from build123d import *

# Parameters (mm, degrees)
ESBO_O1_W                = 150
ESBO_O1_H                = 55
RESSALTO_EXTRUS_O1_DEPTH = 45
FILETE1_R                = 8
ESBO_O2_R                = 3.81
RESSALTO_EXTRUS_O2_DEPTH = 16.806
ESBO_O4_R                = 3.81
RESSALTO_EXTRUS_O3_DEPTH = 16.806


with BuildPart() as part:
    # Esboço1 → Ressalto-extrusão1 (new body)
    with BuildSketch(Plane(origin=(0, 0, 0), x_dir=(1, 0, 0), z_dir=(0, 1, 0))):
        Rectangle(ESBO_O1_W, ESBO_O1_H)
    extrude(amount=RESSALTO_EXTRUS_O1_DEPTH)

    # Filete1
    filete1_edges = [part.edges().sort_by_distance(p)[0] for p in [
        (0, 45, -27.5),
        (0, 0, -27.5),
        (0, 0, 27.5),
        (0, 45, 27.5),
    ]]
    fillet(filete1_edges, radius=FILETE1_R)

    # Esboço2 → Ressalto-extrusão2 (add)
    with BuildSketch(Plane(origin=(0, 0, -27.5), x_dir=(-1, 0, 0), z_dir=(0, 0, -1))):
        with Locations(Location((-68.791943754, 15.581709397, 0), (0, 0, 180))):
            Circle(ESBO_O2_R)
    extrude(amount=RESSALTO_EXTRUS_O2_DEPTH)

    # Esboço4 → Ressalto-extrusão3 (add)
    with BuildSketch(Plane(origin=(0, 0, -27.5), x_dir=(-1, 0, 0), z_dir=(0, 0, -1))):
        with Locations(Location((-68.791943754, 26.164871882, 0), (0, 0, 180))):
            Circle(ESBO_O4_R)
    extrude(amount=RESSALTO_EXTRUS_O3_DEPTH)


solid = part.part
Geometry: final body of the model. Coordinates: model frame, mm. A direction names the side the tool comes from. Coordinates: 2 decimals unless noted, no trailing zeros. Order: outer loops, then holes, each group sorted by start corner. A loop starts at its lowest first (then second) coordinate and runs counter-clockwise, first axis right, second up. Notation, with made-up numbers: M -36,80 L 15,80 A12 cw 15,86 Z; hole C 37.5,-32 d4. An arc over 180 degrees is marked long. One line per question, with ' | ' between items. Start each with the question number.
Item 1: Cut plane B-B, the plane z = -31. Return the cut outline in (x, y), then the cut area to 3 significant figures.
Item 2: Cut plane A-A, the plane x = 43. Return the cut outline in (y, z).
Item 3: Set-up query: faces 1 (the cylindrical face through (72.426, 14.437, -35.785)), 2 (the flat face through (69, 16, -44.306)). Return all of +Z, -Z, +X, -X, +Y, -Y with unobstructed straight access to the full face (end or side cutting, diameter ignored); none if empty.
Item 4: Ray query, probe 1 along Z at (x, y) = (-57, 14); probe 2 along Z at (x, y) = (22, 7); probe 3 along X at (y, z) = (13, -35). Return the intervals inside material, ascending. Write a range as [from, to].
Item 5: Draft query along Y for faces 3 (the cylindrical face through (1.05, 2.406, 25.219)), 4 (the cylindrical face through (72.426, 25.02, -35.785)), 5 (the flat face through (-1, 45, 0)). Return one class per face: released by +Y, released by -Y, zero draft, split by the parting line, or undercut.
Item 6: Cut plane C-C, the plane y = 10. Return the cut outline in (x, z), then the cut area to 3 significant figures.
A:
1) outline: C 68.79,15.58 d7.62; C 68.79,26.16 d7.62 | area: 91.2 mm2
2) outline: M 0,-19.5 A8 ccw 8,-27.5 L 37,-27.5 A8 ccw 45,-19.5 L 45,19.5 A8 ccw 37,27.5 L 8,27.5 A8 ccw 0,19.5 Z
3) face 1: -Z | face 2: -Z, +X, -X, +Y, -Y
4) probe 1: z = [-27.5, 27.5] | probe 2: z = [-27.44, 27.44] | probe 3: x = [65.99, 71.59]
5) face 3: released by -Y | face 4: undercut | face 5: released by +Y
6) outline: M -75,-27.5 L 75,-27.5 L 75,27.5 L -75,27.5 Z | area: 8,250 mm2
